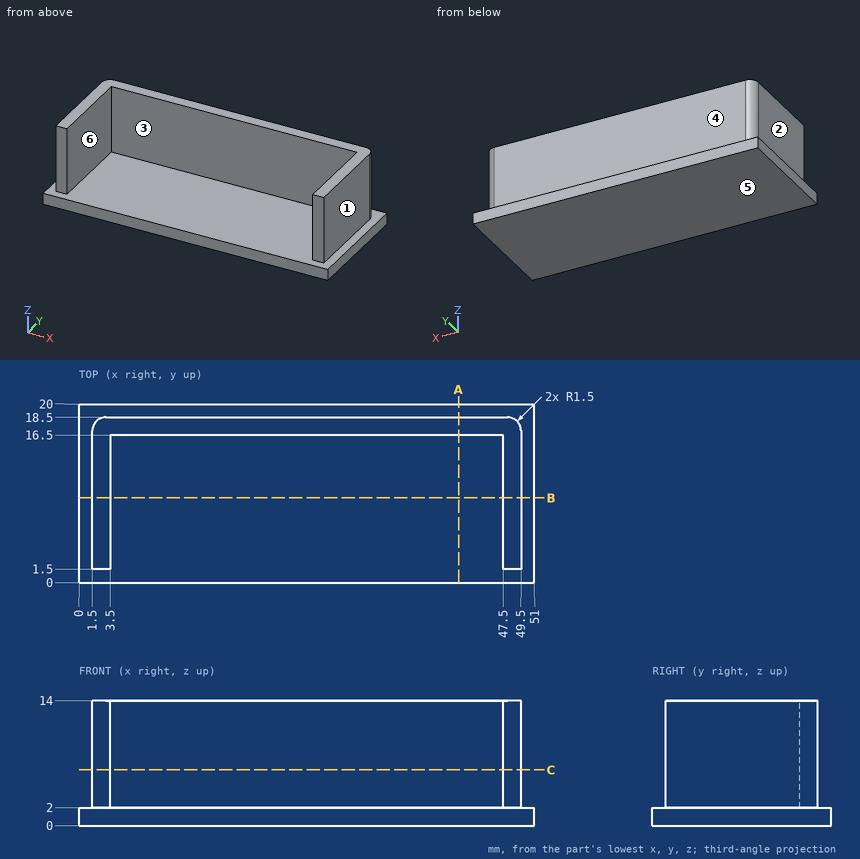
Can you work these out from the drawing? Everything is in mm from the part's minimum corner. A direction names the side the tool comes from. Round coordinates to 2 decimals unless told otherwise and drop trailing zeros. Write each loop counter-clockwise with the first axis right and the second up, starting at its lowest first coordinate (ties: lowest second). Pieces come first, ordered by that corner, then holes. Notation, with made-up numbers: M 10.25,8 L 42.25,8 A29 cw 42.25,33 Z; hole C 57.5,83.5 d1. An arc over 180 degrees is marked long. Use a Markdown table: item, result.
Item 1: I want a section at B-B (y = 9.5). List the corners of the cut face in (x, z) for me, and give its area (3 significant figures).
Found:
| item | result |
|---|---|
| outline | M 0,0 L 51,0 L 51,2 L 49.5,2 L 49.5,14 L 47.5,14 L 47.5,2 L 3.5,2 L 3.5,14 L 1.5,14 L 1.5,2 L 0,2 Z |
| area | 150 mm2 |
Item 2: I want a section at A-A (x = 42.5). List the corners of the cut face in (y, z) for me.
Found:
| item | result |
|---|---|
| outline | M 0,0 L 20,0 L 20,2 L 18.5,2 L 18.5,14 L 16.5,14 L 16.5,2 L 0,2 Z |
Item 3: We'd pull the mould along X, two halves only. Please class the marked faces 1, 2, 3 and 4: released by +X, released by -X, zero draft, split by the parting line, or undercut.
Found:
| item | result |
|---|---|
| face 1 | released by +X |
| face 2 | released by -X |
| face 3 | undercut |
| face 4 | zero draft |
Item 4: Which directions (+Z, -Z, +X, -X, +Y, -Y) give clear straight access to the entire face, cutting with the end or side of a thin tool? Please do the marked faces 5 and 6.
Found:
| item | result |
|---|---|
| face 5 | -Z, +X, -X, +Y, -Y |
| face 6 | +Z, -Y |
Item 5: I want a section at C-C (z = 6.25). List the corners of the cut face in (x, y) for me, and give its area (3 significant figures).
Found:
| item | result |
|---|---|
| outline | M 1.5,1.5 L 3.5,1.5 L 3.5,16.5 L 47.5,16.5 L 47.5,1.5 L 49.5,1.5 L 49.5,17 A1.5 ccw 48,18.5 L 3,18.5 A1.5 ccw 1.5,17 Z |
| area | 155 mm2 |
Item 6: If I drill on line 1 along X through (y, z) = (15.75, 4); line 2 along Y through (x, z) = (29.5, 5.75); line 3 along Z through (x, y) = (5, 11.5), over which ranges is the centre line in solid material (lowest first)? Write a range as [from, to].
Found:
| item | result |
|---|---|
| line 1 | x = [1.5, 3.5], [47.5, 49.5] |
| line 2 | y = [16.5, 18.5] |
| line 3 | z = [0, 2] |
Item 7: For pin 1 Ø1.6 at (x, z) = (49, 8) entering from -Y; pin 2 Ø1 at (y, z) = (14.5, 10) entering from +X; pin 3 Ø10 at (x, y) = (15.5, 10) entering from +Z, each with a flat end and sliding along its axis, tell me the tip position at first contact or that it passes through.
Found:
| item | result |
|---|---|
| pin 1 | stops at y = 1.5 |
| pin 2 | stops at x = 49.5 |
| pin 3 | stops at z = 2 |
